from build123d import *

# Parameters (mm, degrees)
BOSS_EXTRUDE1_DEPTH = 20
BOSS_EXTRUDE2_DEPTH = 4
BOSS_EXTRUDE3_DEPTH = 4
SKETCH4_R           = 2
CUT_EXTRUDE1_DEPTH  = 4
SKETCH5_R           = 2
CUT_EXTRUDE2_DEPTH  = 4


with BuildPart() as part:
    # Sketch1 → Boss-Extrude1 (new body)
    with BuildSketch(Plane.XY):
        Polygon((0, 0), (-20, 0), (-20, 4), (-4, 4), (-4, 20), (0, 20), align=None)
    extrude(amount=BOSS_EXTRUDE1_DEPTH)

    # Sketch2 → Boss-Extrude2 (add)
    with BuildSketch(Plane(origin=(0, 0, 0), x_dir=(-1, 0, 0), z_dir=(0, 0, -1))):
        Polygon((4, 20), (20, 4), (4, 4), align=None)
    extrude(amount=-BOSS_EXTRUDE2_DEPTH)

    # Sketch3 → Boss-Extrude3 (add)
    with BuildSketch(Plane.XY.offset(20)):
        Polygon((-4, 20), (-20, 4), (-4, 4), align=None)
    extrude(amount=-BOSS_EXTRUDE3_DEPTH)

    # Sketch4 → Cut-Extrude1 (cut)
    with BuildSketch(Plane(origin=(0, 4, 0), x_dir=(1, 0, 0), z_dir=(0, 1, 0))):
        with Locations((-12, -10)):
            Circle(SKETCH4_R)
    extrude(amount=-CUT_EXTRUDE1_DEPTH, mode=Mode.SUBTRACT)

    # Sketch5 → Cut-Extrude2 (cut)
    with BuildSketch(Plane.ZY.offset(4)):
        with Locations((10, 12)):
            Circle(SKETCH5_R)
    extrude(amount=-CUT_EXTRUDE2_DEPTH, mode=Mode.SUBTRACT)


solid = part.part
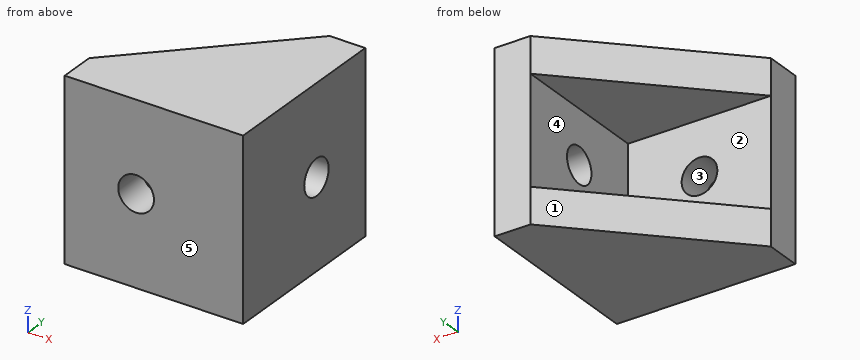
Source: CAD feature listing. Evaluate the final solid. Frame: model axes, mm. Face numbers are marked on the shaded views. A direction names the side the tool comes from. Give positions to 0.01 mm unless a question says otherwise; leave off trailing zeros. Write each loop counter-clockwise with the first axis right and the second up, starting at its lowest first coordinate (ties: lowest second). Pieces come first, ordered by that corner, then holes. Notation, with made-up numbers: M -14,-36.75 L -3,-36.75 A27 ccw -3,-16.75 Z; hole C -40,-4.75 d6. An arc over 180 degrees is marked long. Answer as a JSON object with one key per item and string values.
Q1. Cut plane B-B, the plane y = 12. Return the cut outline in (x, z).
Geometry check:
{"outline": "M -12,0 L 0,0 L 0,8 L -4,8 L -4,4 L -12,4 Z; M -12,16 L -4,16 L -4,12 L 0,12 L 0,20 L -12,20 Z"}
Q2. Contact query for flat-ended pins moving along their axis: P1, Ø5, axis at x = -13.5, y = 16.5, coming from the -Z side; P2, Ø1.5, axis at x = -6.5, z = 6.5, coming from the +Y side; P3, Ø12, axis at x = -10.5, z = 11.5, coming from the +Y side; P4, Ø6, axis at y = 13, z = 12.5, coming from the -X side. Output: stop coordinate, or through.
Geometry check:
{"P1": "passes through", "P2": "stops at y = 4", "P3": "stops at y = 17.47", "P4": "stops at x = -4"}
Q3. Cut plane C-C, the plane z = 10. Return the cut outline in (x, y), then the cut area to 3 significant figures.
Geometry check:
{"outline": "M -20,0 L -14,0 L -14,4 L -20,4 Z; M -10,0 L 0,0 L 0,10 L -4,10 L -4,4 L -10,4 Z; M -4,14 L 0,14 L 0,20 L -4,20 Z", "area": "112 mm^2"}
Q4. Cut plane A-A, the plane x = -12. Return the cut outline in (y, z), then the cut area to 3 significant figures.
Geometry check:
{"outline": "M 0,0 L 12,0 L 12,4 L 4,4 L 4,8 L 0,8 Z; M 0,12 L 4,12 L 4,16 L 12,16 L 12,20 L 0,20 Z", "area": "128 mm^2"}
Q5. Access query for the marked faces 4 and 5. Directions: +Z, -Z, +X, -X, +Y, -Y. A direction counts if a zero-diameter tool reaches every point of the face in a straight line with its end or side. Return the directions, or none.
Geometry check:
{"face 4": "-X, +Y", "face 5": "+Z, -Z, +X, -X, -Y"}
Q6. Ray query, line 1 along X through (y, z) = (2.8, 10); line 2 along Z through (x, y) = (-7, 6.25); line 3 along Z through (x, y) = (-12, 1.45). Return the intervals inside material, ascending.
Geometry check:
{"line 1": "x = -20 to -14, -10 to 0", "line 2": "z = 0 to 4, 16 to 20", "line 3": "z = 0 to 8, 12 to 20"}
Q7. Cut plane D-D, the plane y = 5.5. Return the cut outline in (x, z).
Geometry check:
{"outline": "M -18.5,0 L 0,0 L 0,20 L -18.5,20 L -18.5,16 L -4,16 L -4,4 L -18.5,4 Z"}
Q8. Mould query, pull axis X, two halves, no side actions, for the marked faces 1, 2 and 3. Classes: +X half, -X half, draft (parallel to the pull), parting line (faces both ways), or undercut.
Geometry check:
{"face 1": "-X half", "face 2": "draft", "face 3": "undercut"}
